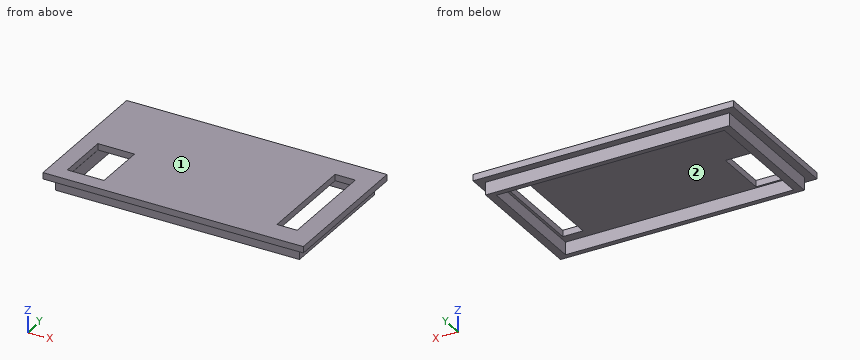
```python
from build123d import *

# Parameters (mm, degrees)
SKETCH003_W     = 41.1
SKETCH003_H     = 23
PAD001_DEPTH    = 1
SKETCH004_W     = 38.5
SKETCH004_H     = 20.6
PAD002_DEPTH    = 2
SKETCH005_W     = 36
SKETCH005_H     = 19
POCKET002_DEPTH = 2.001
SKETCH006_W     = 3.2
SKETCH006_H     = 16
SKETCH006_W_2   = 5.8
SKETCH006_H_2   = 8.4
POCKET003_DEPTH = 1.001


with BuildPart() as part:
    # Sketch003 (on DatumPlane) → Pad001 (new body)
    with BuildSketch(Plane.XY.offset(10.2)):
        Rectangle(SKETCH003_W, SKETCH003_H)
    extrude(amount=PAD001_DEPTH)

    # Sketch004 (on DatumPlane) → Pad002 (join)
    with BuildSketch(Plane.XY.offset(10.2)):
        Rectangle(SKETCH004_W, SKETCH004_H)
    extrude(amount=-PAD002_DEPTH)

    # Sketch005 (on DatumPlane) → Pocket002 (cut, through all)
    with BuildSketch(Plane.XY.offset(10.2)):
        Rectangle(SKETCH005_W, SKETCH005_H)
    extrude(amount=-POCKET002_DEPTH, mode=Mode.SUBTRACT)

    # Sketch006 (on DatumPlane) → Pocket003 (cut, through all)
    with BuildSketch(Plane.XY.offset(10.2)):
        with Locations((15.968977, 0)):
            Rectangle(SKETCH006_W, SKETCH006_H)
        with Locations((-15.127274, -5.017358)):
            Rectangle(SKETCH006_W_2, SKETCH006_H_2)
    extrude(amount=POCKET003_DEPTH, mode=Mode.SUBTRACT)


solid = part.part
```
For this review, take the finished solid that the model builds, in its own axes (mm). Face numbers are marked on the shaded views. Round coordinates to 2 decimals unless told otherwise and drop trailing zeros. Write each loop counter-clockwise with the first axis right and the second up, starting at its lowest first coordinate (ties: lowest second). Pieces come first, ordered by that corner, then holes. Notation, with made-up numbers: (77, -4.5) - (102, -4.5) arc R24 ccw to (102, 30.5) - close; hole circle Ø11 at (26.5, 28.25). An arc over 180 degrees is marked (long way). Write each question's results on one line, items separated by ' | '.
Item 1: Take a section at B-B on x = 16.5. State the section outline as (y, z) points.
Calculated:
outline: (-11.5, 10.2) - (-10.3, 10.2) - (-10.3, 8.2) - (-9.5, 8.2) - (-9.5, 10.2) - (-8, 10.2) - (-8, 11.2) - (-11.5, 11.2) - close; (8, 10.2) - (9.5, 10.2) - (9.5, 8.2) - (10.3, 8.2) - (10.3, 10.2) - (11.5, 10.2) - (11.5, 11.2) - (8, 11.2) - close
Item 2: Take a section at D-D on y = 3.25. State the section outline as (x, z) points, then the cut area to 3 significant figures.
Calculated:
outline: (-20.55, 10.2) - (-19.25, 10.2) - (-19.25, 8.2) - (-18, 8.2) - (-18, 10.2) - (14.37, 10.2) - (14.37, 11.2) - (-20.55, 11.2) - close; (17.57, 10.2) - (18, 10.2) - (18, 8.2) - (19.25, 8.2) - (19.25, 10.2) - (20.55, 10.2) - (20.55, 11.2) - (17.57, 11.2) - close | area: 42.9 mm^2
Item 3: Take a section at A-A on y = -3.25. Count the separate pieces of the cut face and the enclosed holes in it, then the cut area to 3 significant figures.
Calculated:
separate pieces: 3 | enclosed holes: 0 | area: 37.1 mm^2
Item 4: For pin 1 (1 mm diameter, centred on y = 4.5, z = 9.5, fed in from -X); pin 2 (0.6 mm diameter, centred on x = 4, z = 9.5, fed in from -Y); pin 3 (0.6 mm diameter, centred on x = -3, z = 9.5, fed in from +Y), all flat-tipped, find the tip position at first contact; note any pin that passes through.
Calculated:
pin 1: stops at x = -19.25 | pin 2: stops at y = -10.3 | pin 3: stops at y = 10.3
Item 5: To check wall thickness, follow line 1 along Y through (x, z) = (-0.5, 9.5); line 2 along X through (y, z) = (-5, 9.6); line 3 along X through (y, z) = (-0.5, 10.7). State the ranges of each line that lie inside material, in increasing order. Write a range as from..to.
Calculated:
line 1: y = -10.3..-9.5, 9.5..10.3 | line 2: x = -19.25..-18, 18..19.25 | line 3: x = -20.55..14.37, 17.57..20.55
Item 6: Take a section at C-C on z = 10.7. State the section outline as (x, y) points, then the cut area to 3 significant figures.
Calculated:
outline: (-20.55, -11.5) - (20.55, -11.5) - (20.55, 11.5) - (-20.55, 11.5) - close; hole (-18.03, -9.22) - (-12.23, -9.22) - (-12.23, -0.82) - (-18.03, -0.82) - close; hole (14.37, -8) - (17.57, -8) - (17.57, 8) - (14.37, 8) - close | area: 845 mm^2
Item 7: Draft analysis for pull direction Y (two halves, no side actions). For the marked faces 1 and 2, state which applies: pulls with the +Y half, pulls with the -Y half, needs draft (parallel to the pull), parting line crosses it, or undercut.
Calculated:
face 1: needs draft | face 2: undercut
